Can you work these out from the model? Positions are in its coordinate system, mm. A direction names the side the tool comes from. Coordinates: 2 decimals unless noted, no trailing zeros. Order: outer loops, then holes, each group sorted by start corner. A loop starts at its lowest first (then second) coordinate and runs counter-clockwise, first axis right, second up. Notation, with made-up numbers: (83.25, -40) -> (129.25, -40) arc R9 ccw to (129.25, -31) -> close; hole circle Ø6 at (45.25, -13). An arc over 180 degrees is marked (long way). Write item = value, one per line.
```python
from build123d import *

# Parameters (mm, degrees)
CROQUIS1_W              = 40
CROQUIS1_H              = 20.86
CROQUIS1_W_2            = 38
CROQUIS1_H_2            = 18.86
SALIENTE_EXTRUIR1_DEPTH = 120
CROQUIS2_W              = 35
CROQUIS2_H              = 14
CORTAR_EXTRUIR1_DEPTH   = 120


with BuildPart() as part:
    # Croquis1 → Saliente-Extruir1 (new body)
    with BuildSketch(Plane.XY):
        Rectangle(CROQUIS1_W, CROQUIS1_H)
        Rectangle(CROQUIS1_W_2, CROQUIS1_H_2, mode=Mode.SUBTRACT)
    extrude(amount=SALIENTE_EXTRUIR1_DEPTH)

    # Croquis2 → Cortar-Extruir1 (cut)
    with BuildSketch(Plane.ZY.offset(20)):
        with Locations((98.5, 0)):
            Rectangle(CROQUIS2_W, CROQUIS2_H)
    extrude(amount=-CORTAR_EXTRUIR1_DEPTH, mode=Mode.SUBTRACT)


solid = part.part
```
Item 1: I want a section at C-C, the plane x = 5. Please give me the cut outline in (y, z).
A:
outline = (-10.43, 0) -> (-9.43, 0) -> (-9.43, 120) -> (-10.43, 120) -> close; (9.43, 0) -> (10.43, 0) -> (10.43, 120) -> (9.43, 120) -> close
Item 2: I'm going to push a flat-ended pin straight in: P1, Ø0.5, axis at x = -19.5, y = -0.5, coming from the -Z side. Where does the tip first touch, or does it pass through?
A:
P1 = 0
Item 3: For faces 1 (the flat face through (19, 0, 46)), 2 (the flat face through (-2, -10, 120)), which set-ups out of +Z, -Z, +X, -X, +Y, -Y let a thin tool reach every point of the face, with its end or its side?
A:
face_1 = +Z, -Z
face_2 = +Z, +X, -X, +Y, -Y
Item 4: If we mould it in two halves opening along X, with no side actions, what happens to faces 3 (the flat face through (-20, 0, 46)), 4 (the flat face through (-2, -10, 0)), 5 (the flat face through (0, 9.43, 59))? For each: pulls with the +X half, pulls with the -X half, needs draft (parallel to the pull), parting line crosses it, or undercut.
A:
face_3 = pulls with the -X half
face_4 = needs draft
face_5 = undercut
Item 5: I want a section at A-A, the plane y = 4.5. Please give me the cut outline in (x, z), plus the area to 3 significant figures.
A:
outline = (-20, 0) -> (-19, 0) -> (-19, 81) -> (-20, 81) -> close; (-20, 116) -> (-19, 116) -> (-19, 120) -> (-20, 120) -> close; (19, 0) -> (20, 0) -> (20, 81) -> (19, 81) -> close; (19, 116) -> (20, 116) -> (20, 120) -> (19, 120) -> close
area = 170 mm2
Item 6: I want a section at B-B, the plane z = 21. Please give me the cut outline in (x, y), plus the area to 3 significant figures.
A:
outline = (-20, -10.43) -> (20, -10.43) -> (20, 10.43) -> (-20, 10.43) -> close; hole (-19, -9.43) -> (19, -9.43) -> (19, 9.43) -> (-19, 9.43) -> close
area = 118 mm2
Item 7: If I drill on probe 1 along Y at (x, z) = (-11.5, 6); probe 2 along X at (y, z) = (-0.25, 24), over which ranges is the centre line in solid material (lowest first)?
A:
probe_1 = -10.43 to -9.43, 9.43 to 10.43
probe_2 = -20 to -19, 19 to 20
